Input: part model. Units: mm. Frame: model coordinates. Coordinates: 2 decimals unless noted, no trailing zeros. Loops run counter-clockwise (first coordinate to the right, second up) from the corner with the lowest first, then second, coordinate; pieces in that order, holes last.
(1) Section C-C, the plane x = 137. Return loops of the section in (y, z).
(2) Contact query for flat-ended pins moving along their axis: P1, Ø1.5, axis at x = 127.5, y = 20, coming from the +Z side; P2, Ø2, axis at y = 18, z = 4, coming from the +X side; P3, Ø0.8, axis at x = 123, z = 4, coming from the -Y side. Output: stop coordinate, or through.
(3) Section A-A, the plane z = 2.05. Return loops of the section in (x, y), then the cut area to 3 significant figures.
(4) Section B-B, the plane y = 25.5. Return loops of the section in (x, z), then the cut area to 3 significant figures.
(5) Line query: L1, parallel to X at y = 15.25, z = 3.55; L2, parallel to Y at x = 135, z = 4.45; L3, parallel to X at y = 15.25, z = 1.1. Output: solid intervals per line, ascending.
```python
from build123d import *

# Parameters (mm, degrees)
EXTRUSION1_DEPTH = 6
ESQUISSE2_R      = 0.2
EXTRUSION2_DEPTH = 20


with BuildPart() as part:
    # Esquisse1 → Extrusion1 (new body)
    with BuildSketch(Plane.XY):
        Polygon((123.733692342, 14.5), (123.733692342, 31.5), (143.838461576, 31.5), (143.838461576, 33.5), (122.759551823, 33.5), (122.759551823, 14.5), align=None)
    extrude(amount=EXTRUSION1_DEPTH)

    # Esquisse2 → Extrusion2 (add)
    with BuildSketch(Plane.XZ.offset(-31.5)):
        with Locations((128.735391716, 4.056660757)):
            Circle(ESQUISSE2_R)
        with Locations((128.971557812, 1.159084415)):
            Circle(ESQUISSE2_R)
    extrude(amount=EXTRUSION2_DEPTH)


solid = part.part
```
Report:
1. outline: (31.5, 0) - (33.5, 0) - (33.5, 6) - (31.5, 6) - close
2. P1: passes through
2. P2: stops at x = 128.94
2. P3: stops at y = 14.5
3. outline: (122.76, 14.5) - (123.73, 14.5) - (123.73, 31.5) - (143.84, 31.5) - (143.84, 33.5) - (122.76, 33.5) - close
3. area: 58.7 mm2
4. outline: (122.76, 0) - (123.73, 0) - (123.73, 6) - (122.76, 6) - close; circle Ø0.4 at (128.74, 4.06); circle Ø0.4 at (128.97, 1.16)
4. area: 6.10 mm2
5. L1: x = 122.76 to 123.73
5. L2: y = 31.5 to 33.5
5. L3: x = 122.76 to 123.73, 128.78 to 129.16
